Part print with two shaded views. Sizes in mm from the minimum x, y, z corner. A direction names the side the tool comes from. Give positions to 0.01 mm unless a question says otherwise; leave off trailing zeros. Write each loop counter-clockwise with the first axis right and the second up, starting at its lowest first coordinate (ties: lowest second). Pieces come first, ordered by that corner, then holes.
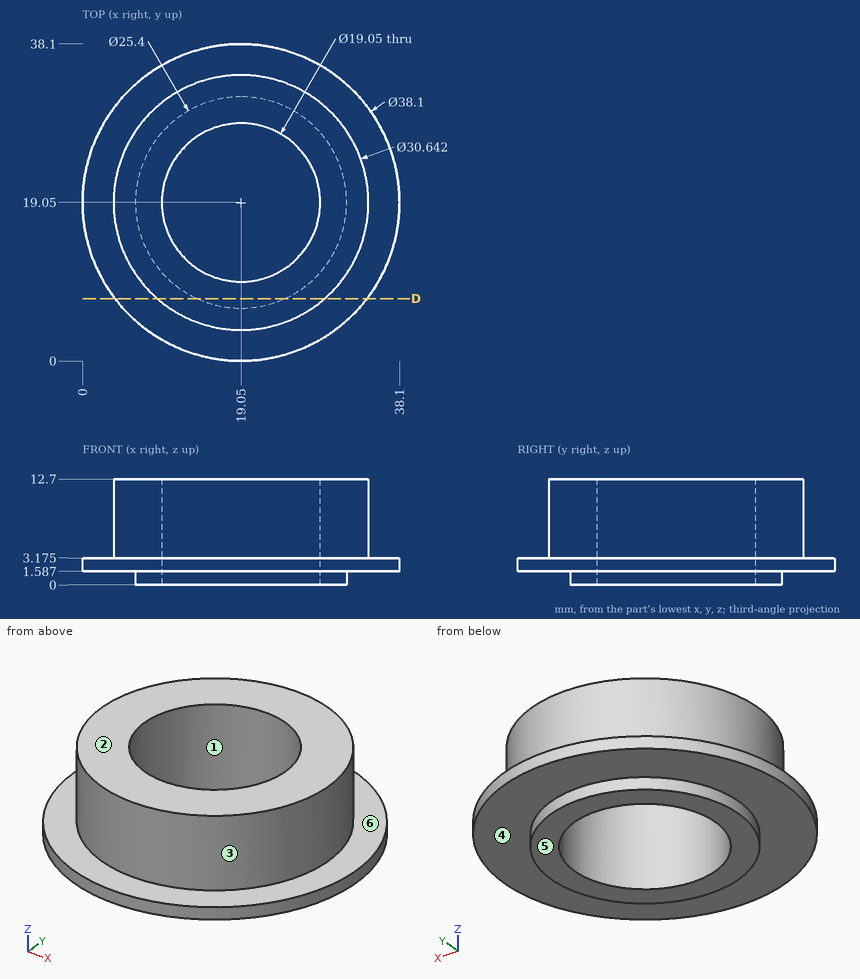
1) Flat gauge pins, fed straight in: P1, Ø1.5, axis at y = 25, z = 5, coming from the +X side; P2, Ø1, axis at x = 8.5, z = 5.5, coming from the -Y side (1 decimal); P3, Ø1.5, axis at x = 30, z = 7.5, coming from the +Y side. Where does each tip first touch, or does it go through?
Check result:
P1: stops at x = 33.46
P2: stops at y = 7.5
P3: stops at y = 30.48
2) Drill centre lines: L1, parallel to Y at x = 19.05, z = 5.75 (1 decimal); L2, parallel to X at y = 22, z = 1; L3, parallel to Z at x = 16.5, y = 3.5 (1 decimal). Where is each one in solid material? Low to high.
Check result:
L1: y = 3.7 to 9.5, 28.6 to 34.4
L2: x = 6.7 to 9.99, 28.11 to 31.4
L3: z = 1.6 to 3.2
3) Mould opens along Y. For the marked faces 1, 2 and 3 say: +Y half, -Y half, draft (parallel to the pull), parting line (faces both ways), or undercut.
Check result:
face 1: undercut
face 2: draft
face 3: parting line
4) Saw through at D-D (y = 7.5). Write the cut outline in (x, z) (1 decimal), and give its area (3 significant figures).
Check result:
outline: (3.9, 1.6) - (13.8, 1.6) - (13.8, 0) - (24.3, 0) - (24.3, 1.6) - (34.2, 1.6) - (34.2, 3.2) - (29.1, 3.2) - (29.1, 12.7) - (9, 12.7) - (9, 3.2) - (3.9, 3.2) - close
area: 257 mm2
5) 3-axis set-ups, long thin cutter, end or side, ignore diameter. For the marked faces 4, 5 and 6: which of +Z, -Z, +X, -X, +Y, -Y reach the whole face in a straight line?
Check result:
face 4: -Z
face 5: -Z, +X, -X, +Y, -Y
face 6: +Z
